Autodesk Inventor part; units mm, degrees
ref_plane "YZ Plane" through (0, 0, 0) normal (1, 0, 0) x (0, 1, 0)
ref_plane "XZ Plane" through (0, 0, 0) normal (0, 1, 0) x (-1, 0, 0)
ref_plane "XY Plane" through (0, 0, 0) normal (0, 0, 1) x (1, 0, 0)
ref_plane "Work Plane1" through (0, 0, 0) normal (0, 0, 1) x (1, 0, 0)
sketch "Sketch1" plane through (0, 0, 0) normal (0, 0, 1) x (1, 0, 0)
  circle A0 centre (-10.1084, -16.6095) radius 3 construction
  circle A1 centre (-10.1084, -56.6095) radius 3 construction
  circle A2 centre (-10.1084, -36.6095) radius 5.15
  line L0 (-29.1084, -220.5) -> (-29.1084, 29.5)
  line L1 (-35.1084, -220.5) -> (-35.1084, 29.5)
  line L2 (-40.1084, -61.6095) -> (-5.1084, -61.6095)
  line L3 (-5.1084, -61.6095) -> (-5.1084, -11.6095)
  line L4 (-5.1084, -11.6095) -> (-40.1084, -11.6095)
  line L5 (-40.1084, -11.6095) -> (-40.1084, -61.6095)
  line L6 (-40.1084, -61.6095) -> (-5.1084, -11.6095) construction
  line L7 (-5.1084, -61.6095) -> (-40.1084, -11.6095) construction
  circle A3 centre (-10.1084, -16.6095) radius 3.1
  circle A4 centre (-10.1084, -56.6095) radius 3.1
  point P0 (0, 0)
  point P1 (-22.6084, -36.6095)
  point P2 (-5.1084, -35.3756)
  point P3 (-5.1084, -37.8434)
  dimension "d0" = 35
  dimension "d1" = 50
  dimension "d2" = 5
  dimension "d3" = 6.2
  dimension "d4" = 6.2
extrude "Extrusion1" add sketch "Sketch1" along normal mid plane 16 contours A2 L3 L2 L0 L4 | L0 L2 L1 L4 | L1 L2 L5 L4
sketch "Sketch2" plane through (-40.1084, -61.6095, 8) normal (0, -1, 0) x (1, 0, 0)
  circle A0 centre (8, -8) radius 6
  circle A1 centre (8, -8) radius 6.3
  point P0 (40.1084, -8)
  dimension "d7" = 0.3
extrude "Extrusion2" cut sketch "Sketch2" against normal through all contours A0 | A1
chamfer "Chamfer1" distance 4 angle 45 4 edges at (-5.1084, -61.6095, 0) (-5.1084, -11.6095, 0) (-40.1084, -61.6095, 0) (-40.1084, -11.6095, 0)
properties part number "06_OPENTRONS_Microscope_Extraslide_slide"
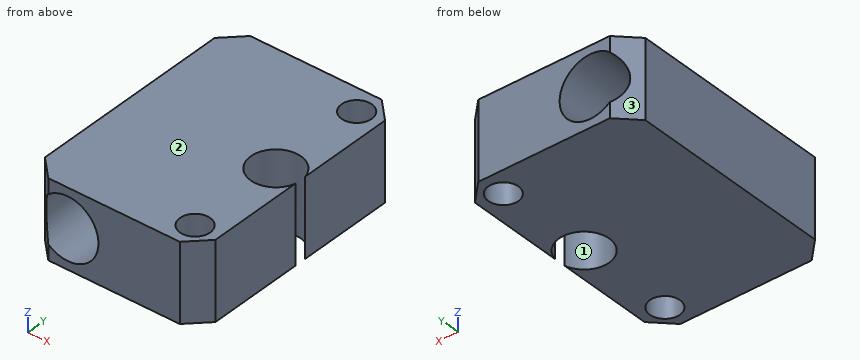
Geometry check sheet. Reference: the model listing, model coordinates, mm. Face numbers are marked on the shaded views. Coordinates: 2 decimals unless noted, no trailing zeros. Loops run counter-clockwise (first coordinate to the right, second up) from the corner with the lowest first, then second, coordinate; pieces in that order, holes last. Notation, with made-up numbers: (68.5, 43.25) - (99.5, 43.25) arc R17 cw to (99.5, 73.25) - close; hole circle Ø6 at (76, -18.5). An arc over 180 degrees is marked (long way). One line per item, written item: value. Start each with the question number.
(1) Cross-section at A-A on z = -3.5. Enter the section's corners in (x, y), plus the area to 3 significant figures.
(2) Mould release check, pull along Y, two halves, no side actions. Record for the marked faces 1, 2 and 3: released by +Y, released by -Y, zero draft, split by the parting line, or undercut.
(3) Depth check by flat-ended pin: P1, Ø9.5, axis at x = -10.11, y = -36.61, coming from the +Z side. Enter the tip coordinate at first touch or a pass-through.
(4) Cross-section at C-C on x = -10.5. Enter the section's corners in (y, z), plus the area to 3 significant figures.
(5) Material ranges on line 1 (X direction, y = -14, z = -5.5); line 2 (X direction, y = -59, z = 5.5); line 3 (Y direction, x = -11.5, z = -5), recorded low to high. Write a range as [from, to].
(6) Cross-section at D-D on y = -51. Enter the section's corners in (x, z).
(7) Cross-section at B-B on y = -39. Enter the section's corners in (x, z).
Results below:
1. outline: (-40.11, -57.61) - (-37.35, -60.37) - (-37.35, -12.85) - (-40.11, -15.61) - close; (-26.87, -61.61) - (-9.11, -61.61) - (-5.11, -57.61) - (-5.11, -37.84) arc R5.15 cw (long way) to (-5.11, -35.38) - (-5.11, -15.61) - (-9.11, -11.61) - (-26.87, -11.61) - close; hole circle Ø6.2 at (-10.11, -56.61); hole circle Ø6.2 at (-10.11, -16.61)
1. area: 1,050 mm2
2. face 1: undercut
2. face 2: zero draft
2. face 3: released by +Y
3. P1: passes through
4. outline: (-61.61, -8) - (-59.68, -8) - (-59.68, 8) - (-61.61, 8) - close; (-53.53, -8) - (-41.74, -8) - (-41.74, 8) - (-53.53, 8) - close; (-31.47, -8) - (-19.68, -8) - (-19.68, 8) - (-31.47, 8) - close; (-13.53, -8) - (-11.61, -8) - (-11.61, 8) - (-13.53, 8) - close
4. area: 439 mm2
5. line 1: x = [-38.5, -35.18], [-29.04, -11.78], [-8.43, -6.72]
5. line 2: x = [-38.72, -35.18], [-29.04, -12.08], [-8.13, -6.5]
5. line 3: y = [-61.61, -59.38], [-53.84, -41.57], [-31.65, -19.38], [-13.84, -11.61]
6. outline: (-40.11, -8) - (-5.11, -8) - (-5.11, 8) - (-40.11, 8) - close; hole circle Ø12.6 at (-32.11, 0)
7. outline: (-40.11, -8) - (-14.67, -8) - (-14.67, 8) - (-40.11, 8) - close; (-5.55, -8) - (-5.11, -8) - (-5.11, 8) - (-5.55, 8) - close; hole circle Ø12.6 at (-32.11, 0)
